Source: CAD feature listing. Evaluate the final solid. Frame: model axes, mm. Round coordinates to 2 decimals unless told otherwise and drop trailing zeros. Loops run counter-clockwise (first coordinate to the right, second up) from the corner with the lowest first, then second, coordinate; pieces in that order, holes last. Notation, with made-up numbers: M 9.5,18.5 L 54.5,18.5 A9 cw 54.5,31.5 Z; hole C 41.25,84.25 d5. An arc over 180 degrees is marked long. Write each question's results on one line, items separated by ' | '. Start each with the question number.
1. Ray query, line 1 (Y direction, x = 33.2, z = -153.74) (1 decimal); line 2 (Y direction, x = 32.5, z = -26); line 3 (Y direction, x = 33.55, z = -90.5). Return the intervals inside material, ascending.
2. Contact query for flat-ended pins moving along their axis: pin 1 Ø9 at (y, z) = (140.46, -102.94) entering from +X; pin 2 Ø0.8 at (x, z) = (33.5, 21) entering from -Y; pin 3 Ø0.5 at (x, z) = (33.5, 26) entering from +Y. Output: stop coordinate, or through.
3. Section A-A on z = -141.04. Output: boundary loops of the cut face in (x, y).
4. Draft query along Y for faces 1 (the flat face through (33.201, 117.721, -165.596)), 2 (the cylindrical face through (33.201, 135.117, -69.252)), 3 (the flat face through (33.201, 172.822, -117.633)). Return one class per face: released by +Y, released by -Y, zero draft, split by the parting line, or undercut.
5. Section D-D on x = 33.1. Give the number of separate pieces and of enclosed holes in the cut face, and give its area (3 significant figures).
6. Section C-C on z = -115.64. Output: boundary loops of the cut face in (x, y) (3 decimals).
7. Section B-B on y = 115. Output: boundary loops of the cut face in (x, z).
Autodesk Inventor part; units mm, degrees
ref_plane "YZ Plane" through (0, 0, 0) normal (1, 0, 0) x (0, 1, 0)
ref_plane "XZ Plane" through (0, 0, 0) normal (0, 1, 0) x (-1, 0, 0)
ref_plane "XY Plane" through (0, 0, 0) normal (0, 0, 1) x (1, 0, 0)
ref_plane "Work Plane1" through (32.4184, 134.1094, 24.06) normal (1, 0, 0) x (0, 1, 0)
sketch "Sketch1" plane through (32.4184, 134.1094, 24.06) normal (1, 0, 0) x (0, 1, 0)
  line L0 (-24.13, 172.2574) -> (-24.13, 6.35)
  line L1 (-24.13, 6.35) -> (-2.1844, 6.35)
  line L2 (-10.3187, -184.15) -> (-2.3114, -184.15)
  circle A0 centre (6.35, -127) radius 2.1844
  circle A1 centre (6.35, -38.1) radius 2.1844
  circle A2 centre (0, -82.55) radius 2.1844
  circle A3 centre (0, 6.35) radius 2.1844
  circle A4 centre (0, -6.35) radius 2.1844
  circle A5 centre (42.3182, -89.0797) radius 2.1844
  line L3 (-24.13, 6.35) -> (-24.13, -179.6761)
  line L4 (-22.1107, -184.3202) -> (-10.5035, -195.1441)
  line L5 (-6.1728, -196.85) -> (22.906, -196.85)
  line L6 (29.1428, -191.6937) -> (48.555, -90.2734)
  line L7 (-24.13, 6.35) -> (12.7, 6.35)
  line L8 (12.7, -7.2898) -> (12.7, -68.7578)
  circle A6 centre (42.3182, -89.0797) radius 6.35
  line L9 (48.0429, -86.3318) -> (15.2013, -17.911)
  line L10 (12.7, -6.9198) -> (12.7, 6.35)
  circle A7 centre (21.8059, -177.8) radius 2.1844
  circle A8 centre (21.8059, -165.1) radius 2.1844
  arc A9 (12.7, -6.9198) -> (15.2013, -17.911) centre (38.1, -6.9198) ccw
  arc A10 (22.906, -196.85) -> (29.1428, -191.6937) centre (22.906, -190.5) ccw
  arc A11 (-10.5035, -195.1441) -> (-6.1728, -196.85) centre (-6.1728, -190.5) ccw
  arc A12 (-24.13, -179.6761) -> (-22.1107, -184.3202) centre (-17.78, -179.6761) ccw
  circle A13 centre (-6.35, -76.2) radius 2.1844 construction
  line L11 (-24.13, -22.86) -> (-24.13, -50.8) construction
  line L12 (-24.13, -50.8) -> (-36.83, -76.2) construction
  line L13 (-36.83, -76.2) -> (-24.13, -101.6) construction
  line L14 (-24.13, -101.6) -> (-24.13, -129.54) construction
  spline S0 degree 4 poles (-24.13, -22.86) (-24.13, -50.8) (-36.83, -76.2) (-24.13, -101.6) (-24.13, -129.54) knots 1 1 1 1 1 2 2 2 2 2
  circle A14 centre (6.35, -127) radius 4.953
  circle A15 centre (6.35, -38.1) radius 4.953
  circle A16 centre (0, -95.25) radius 2.1844
  circle A17 centre (6.35, -25.4) radius 2.1844
  circle A18 centre (6.35, -50.8) radius 2.1844
  circle A19 centre (0, -95.25) radius 2.1844
  circle A20 centre (0, -69.85) radius 2.1844
  circle A21 centre (0, -82.55) radius 2.1844
  circle A22 centre (6.35, -114.3) radius 2.1844
  circle A23 centre (6.35, -139.7) radius 2.1844
  circle A24 centre (6.35, -127) radius 2.1844
  circle A25 centre (-6.35, -177.8) radius 2.1844
  point P0 (-134.1094, -24.06)
  point P1 (0, -82.55)
  point P2 (-8.6741, -196.85)
  point P3 (28.1559, -196.85)
  point P4 (12.7, -12.7)
  point P5 (-6.3151, -184.15)
  point P6 (2.1844, 6.35)
  point P7 (-24.13, -22.86)
  point P8 (-24.13, -129.54)
  dimension "d0" = 12.7
  dimension "d1" = 12.7
  dimension "d2" = 133
  dimension "d3" = 6.35
  dimension "d4" = 36.83
  dimension "d5" = 19.05
  dimension "d6" = 25.4
  dimension "d7" = 6.35
  dimension "d8" = 27.94
  dimension "d9" = 27.94
  dimension "d10" = 25.4
  dimension "d11" = 25.4
  dimension "d12" = 12.7
  dimension "d13" = 9.906
  dimension "d14" = 9.906
  dimension "d18" = 4.3688
extrude "Extrusion1" add sketch "Sketch1" along normal blind 1.5875 contours L1 A3 L7 L10 A9 L9 A6 L6 A10 L5 A11 L4 A12 L3 | L3 S0 | A6
Taken from the geometry:
1) line 1: 110 to 125.6, 129.9 to 153.7, 158.1 to 165.9 | line 2: 107.29 to 138.4, 142.51 to 164.74 | line 3: 108.92 to 138.29, 142.63 to 178.02
2) pin 1: through | pin 2: y = 109.98 | pin 3: y = 146.81
3) outline: M 32.42,109.98 L 34.01,109.98 L 34.01,153.73 L 32.42,153.73 Z; M 32.42,158.1 L 34.01,158.1 L 34.01,168.34 L 32.42,168.34 Z
4) face 1: released by -Y | face 2: undercut | face 3: released by +Y
5) separate pieces: 1 | enclosed holes: 14 | area: 11,500 mm^2
6) outline: M 32.418,109.979 L 34.006,109.979 L 34.006,138.275 L 32.418,138.275 Z; M 32.418,142.644 L 34.006,142.644 L 34.006,173.204 L 32.418,173.204 Z
7) outline: M 32.42,-163.06 L 34.01,-163.06 L 34.01,30.41 L 32.42,30.41 Z
